```python
from build123d import *

# Parameters (mm, degrees)
BOSS_EXTRUDE1_DEPTH = 11
BOSS_EXTRUDE2_DEPTH = 17
BOSS_EXTRUDE3_DEPTH = 10
SKETCH4_R           = 11
BOSS_EXTRUDE4_DEPTH = 2


with BuildPart() as part:
    # Sketch1 → Boss-Extrude1 (new body)
    with BuildSketch(Plane(origin=(0, 0, 0), x_dir=(1, 0, 0), z_dir=(0, 1, 0))):
        Polygon((19.15, -21.15), (21.15, -19.15), (21.15, 19.15), (19.15, 21.15), (-19.15, 21.15), (-21.15, 19.15), (-21.15, -19.15), (-19.15, -21.15), align=None)
    extrude(amount=BOSS_EXTRUDE1_DEPTH)

    # Sketch2 → Boss-Extrude2 (add)
    with BuildSketch(Plane(origin=(0, 11, 0), x_dir=(1, 0, 0), z_dir=(0, 1, 0))):
        Polygon((16.15, -21.15), (21.15, -16.15), (21.15, 16.15), (16.15, 21.15), (-16.15, 21.15), (-21.15, 16.15), (-21.15, -16.15), (-16.15, -21.15), align=None)
    extrude(amount=BOSS_EXTRUDE2_DEPTH)

    # Sketch3 → Boss-Extrude3 (add)
    with BuildSketch(Plane(origin=(0, 28, 0), x_dir=(1, 0, 0), z_dir=(0, 1, 0))):
        Polygon((19.15, -21.15), (21.15, -19.15), (21.15, 19.15), (19.15, 21.15), (-19.15, 21.15), (-21.15, 19.15), (-21.15, -19.15), (-19.15, -21.15), align=None)
    extrude(amount=BOSS_EXTRUDE3_DEPTH)

    # Sketch4 → Boss-Extrude4 (add)
    with BuildSketch(Plane(origin=(0, 38, 0), x_dir=(1, 0, 0), z_dir=(0, 1, 0))):
        with Locations(Location((0, 0, 0), (0, 0, 270))):
            Circle(SKETCH4_R)
    extrude(amount=BOSS_EXTRUDE4_DEPTH)


solid = part.part
```
For this review, take the finished solid that the model builds, in its own axes (mm). A direction names the side the tool comes from. Round coordinates to 2 decimals unless told otherwise and drop trailing zeros. Write each loop counter-clockwise with the first axis right and the second up, starting at its lowest first coordinate (ties: lowest second). Pieces come first, ordered by that corner, then holes.
1) Machinability: for faces 1 (the face through (18.7, 19.4, -18.6)), 2 (the face through (-10, 38, 9)), 3 (the face through (19, 11, 19)), 4 (the face through (-20.2, 5.4, 20.1)), 5 (the face through (-19, 11, 19)), which of the approach directions +Z, -Z, +X, -X, +Y, -Y give a long, thin tool a straight path to every point of the face, cutting with its end or side? Answer none if there is none.
Answer below:
face 1: -Z, +X
face 2: +Y
face 3: +Z, +X
face 4: +Z, -X, +Y, -Y
face 5: +Z, -X
2) Mouldability with a two-part tool opening along Y and no side actions: class faces 6 (the face through (19, 11, -19)), 7 (the face through (21.15, 19, 0)), 8 (the face through (0, 40, 0)) as +Y half, -Y half, draft (parallel to the pull), parting line (faces both ways), or undercut.
Answer below:
face 6: undercut
face 7: draft
face 8: +Y half
3) Take a section at D-D on x = 17. Give the boundary of the cut face in (y, z), then the cut area to 3 significant figures.
Answer below:
outline: (0, -21.15) - (11, -21.15) - (11, -20.3) - (28, -20.3) - (28, -21.15) - (38, -21.15) - (38, 21.15) - (28, 21.15) - (28, 20.3) - (11, 20.3) - (11, 21.15) - (0, 21.15) - close
area: 1,580 mm2
4) Take a section at C-C on z = -17.5. Give the boundary of the cut face in (x, y), then the cut area to 3 significant figures.
Answer below:
outline: (-21.15, 0) - (21.15, 0) - (21.15, 11) - (19.8, 11) - (19.8, 28) - (21.15, 28) - (21.15, 38) - (-21.15, 38) - (-21.15, 28) - (-19.8, 28) - (-19.8, 11) - (-21.15, 11) - close
area: 1,560 mm2
5) For line 1 along Y through (x, z) = (-14.5, 5.5); line 2 along Z through (x, y) = (19, 18); line 3 along X through (y, z) = (20, 19.5), list the stretches that pass through material, from the lowest coordinate up.
Answer below:
line 1: y = 0 to 38
line 2: z = -18.3 to 18.3
line 3: x = -17.8 to 17.8
6) Insertion check: pin 1 Ø4 at (x, z) = (-19, 17.5) entering from +Y. The pin has a flat end and moves straight along its axis. Give the tip position at first contact, or say it passes through.
Answer below:
pin 1: stops at y = 38
7) Take a section at B-B on y = 16. Give the boundary of the cut face in (x, z).
Answer below:
outline: (-21.15, -16.15) - (-16.15, -21.15) - (16.15, -21.15) - (21.15, -16.15) - (21.15, 16.15) - (16.15, 21.15) - (-16.15, 21.15) - (-21.15, 16.15) - close
8) Take a section at A-A on x = 0. Give the boundary of the cut face in (y, z).
Answer below:
outline: (0, -21.15) - (38, -21.15) - (38, -11) - (40, -11) - (40, 11) - (38, 11) - (38, 21.15) - (0, 21.15) - close
